from build123d import *

# Parameters (mm, degrees)
SKETCH_1_W      = 2.4
SKETCH_1_H      = 2.4
EXTRUDE_1_DEPTH = 11.5
SKETCH_2_R      = 0.235
EXTRUDE_2_DEPTH = 3.25
SKETCH_3_R      = 0.235
EXTRUDE_3_DEPTH = 3.25


with BuildPart() as part:
    # ｽｹｯﾁ1 → ﾎﾞｽ - 押し出し1 (new body)
    with BuildSketch(Plane.XY):
        with Locations((1.2, 1.2)):
            Rectangle(SKETCH_1_W, SKETCH_1_H)
    extrude(amount=EXTRUDE_1_DEPTH)

    # ｽｹｯﾁ2 → ﾎﾞｽ - 押し出し2 (add)
    with BuildSketch(Plane.XY.offset(11.5)):
        with Locations((1.2, 1.2)):
            Circle(SKETCH_2_R)
    extrude(amount=EXTRUDE_2_DEPTH)

    # ｽｹｯﾁ3 → ﾎﾞｽ - 押し出し3 (add)
    with BuildSketch(Plane(origin=(0, 0, 0), x_dir=(-1, 0, 0), z_dir=(0, 0, -1))):
        with Locations((-1.2, 1.2)):
            Circle(SKETCH_3_R)
    extrude(amount=EXTRUDE_3_DEPTH)


solid = part.part
The listing builds one solid part. Answer for the finished solid, in the listing's coordinates (mm). Coordinates: 2 decimals unless noted, no trailing zeros. Loops run counter-clockwise (first coordinate to the right, second up) from the corner with the lowest first, then second, coordinate; pieces in that order, holes last.
1) Find section A-A on y = 1.2. Write down the section's boundary in (x, z) (3 decimals).
2) Find the intervals of material crossed by L1, parallel to Z at x = 1.65, y = 0.8; L2, parallel to X at y = 1.15, z = -1, in increasing order.
3) Determine the mould class of faces 1 (the face through (1, 0, 6)), 2 (the face through (1, 2.4, 6)), 3 (the face through (2.4, 1, 6)) for opening direction Y: pulls with the +Y half, pulls with the -Y half, needs draft (parallel to the pull), parting line crosses it, or undercut.
4) A flat-ended cylindrical pin translates along its axis: pin 1 Ø1 at (x, y) = (1, 2) entering from +Z. Find the tip coordinate at first contact, or state that the pin passes through.
Values:
1. outline: (0, 0) - (0.965, 0) - (0.965, -3.25) - (1.435, -3.25) - (1.435, 0) - (2.4, 0) - (2.4, 11.5) - (1.435, 11.5) - (1.435, 14.75) - (0.965, 14.75) - (0.965, 11.5) - (0, 11.5) - close
2. L1: z = 0 to 11.5
2. L2: x = 0.97 to 1.43
3. face 1: pulls with the -Y half
3. face 2: pulls with the +Y half
3. face 3: needs draft
4. pin 1: stops at z = 11.5
